The model under review builds one solid part; all positions refer to its coordinate system, in mm. Face numbers are marked on the shaded views. A direction names the side the tool comes from. Give positions to 0.01 mm unless a question says otherwise; leave off trailing zeros. Loops run counter-clockwise (first coordinate to the right, second up) from the corner with the lowest first, then second, coordinate; pieces in that order, holes last. Notation, with made-up numbers: M 76,-31 L 133,-31 A14 cw 133,-23 Z; hole C -5.75,68 d9. An arc over 180 degrees is marked long. Return JSON: item names as keys, results as strings.
Autodesk Inventor part; units mm, degrees
ref_plane "YZ Plane" through (0, 0, 0) normal (1, 0, 0) x (0, 1, 0)
ref_plane "XZ Plane" through (0, 0, 0) normal (0, 1, 0) x (-1, 0, 0)
ref_plane "XY Plane" through (0, 0, 0) normal (0, 0, 1) x (1, 0, 0)
sketch "Sketch1" plane through (0, 0, 0) normal (0, 0, 1) x (1, 0, 0)
  line L0 (0, 0) -> (47, 0)
  line L1 (51, 4) -> (51, 33)
  line L2 (47, 37) -> (0, 37)
  line L3 (0, 37) -> (0, 0)
  circle A0 centre (42, 18.5) radius 4.25
  line L4 (47, 37) -> (51, 33)
  line L5 (47, 0) -> (51, 4)
  line L6 (10, 34) -> (16, 34)
  line L7 (16, 34) -> (16, 26)
  line L8 (16, 26) -> (10, 26)
  line L9 (10, 26) -> (10, 34)
  line L10 (10, 11) -> (16, 11)
  line L11 (16, 11) -> (16, 3)
  line L12 (16, 3) -> (10, 3)
  line L13 (10, 3) -> (10, 11)
  line L14 (10, 26) -> (16, 11) construction
  line L15 (10, 11) -> (16, 26) construction
  circle A1 centre (42, 18.5) radius 16 construction
  line L16 (24, 37) -> (24, 0) construction
  point P0 (51, 37)
  point P1 (51, 0)
  point P2 (0, 18.5)
  point P3 (13, 18.5)
  dimension "d0" = 4
  dimension "d1" = 4
  dimension "d2" = 4
  dimension "d3" = 4
  dimension "d4" = 8.5
  dimension "d5" = 37
  dimension "d6" = 6
  dimension "d7" = 8
  dimension "d8" = 8
  dimension "d9" = 15
  dimension "d10" = 10
  dimension "d11" = 32
  dimension "d12" = 9
  dimension "d13" = 26
  dimension "d14" = 24
extrude "Extrusion1" add sketch "Sketch1" along normal blind 6
sketch "Sketch2" plane through (0, 0, 6) normal (0, 0, 1) x (1, 0, 0)
  line L0 (16, 26) -> (10, 26)
  line L1 (0, 37) -> (0, 0)
  line L2 (0, 34) -> (-4, 34)
  line L3 (-6, 32) -> (-6, 28)
  line L4 (-4, 26) -> (0, 26)
  line L5 (0, 26) -> (0, 34)
  line L6 (0, 11) -> (-4, 11)
  line L7 (-6, 9) -> (-6, 5)
  line L8 (-4, 3) -> (0, 3)
  line L9 (0, 3) -> (0, 11)
  arc A0 (-4, 34) -> (-6, 32) centre (-4, 32) ccw
  arc A1 (-6, 28) -> (-4, 26) centre (-4, 28) ccw
  arc A2 (-4, 11) -> (-6, 9) centre (-4, 9) ccw
  arc A3 (-6, 5) -> (-4, 3) centre (-4, 5) ccw
  dimension "d17" = 2
  dimension "d18" = 6
  dimension "d19" = 8
  dimension "d20" = 8
  dimension "d21" = 15
extrude "Extrusion2" add sketch "Sketch2" against normal blind 6
properties part number "y_carriage_belt_iddler"
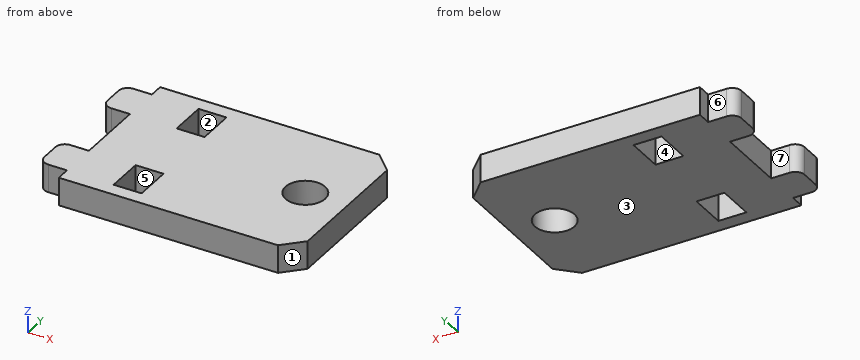
1) Tool access review of the marked faces 5, 6 and 7: name each direction out of +Z, -Z, +X, -X, +Y, -Y from which nothing blocks a thin tool from reaching the whole face with its end or side.
From the geometry:
{"face 5": "+Z, -Z", "face 6": "+Z, -Z, -X, +Y", "face 7": "+Z, -Z, -X"}
2) Consider section D-D on y = 13.5. Write out the cut boundary in (x, z).
From the geometry:
{"outline": "M 0,0 L 51,0 L 51,6 L 0,6 Z"}
3) Insertion check: pin 1 (0.9 mm diameter, centred on y = 1, z = 4, fed in from -X); pin 2 (2.5 mm diameter, centred on y = 35, z = 3.5, fed in from -X); pin 3 (1.2 mm diameter, centred on x = -1.5, z = 3.5, fed in from +Y). Each pin has a flat end and moves straight along its axis. Give the tip position at first contact, or say it passes through.
From the geometry:
{"pin 1": "x = 0", "pin 2": "x = -4.97", "pin 3": "y = 34"}
4) Consider section B-B on z = 5.25. Write out the cut boundary in (x, y).
From the geometry:
{"outline": "M -6,5 A2 ccw -4,3 L 0,3 L 0,0 L 47,0 L 51,4 L 51,33 L 47,37 L 0,37 L 0,34 L -4,34 A2 ccw -6,32 L -6,28 A2 ccw -4,26 L 0,26 L 0,11 L -4,11 A2 ccw -6,9 Z; hole M 10,3 L 16,3 L 16,11 L 10,11 Z; hole M 10,26 L 16,26 L 16,34 L 10,34 Z; hole C 42,18.5 d8.5"}
5) Wall thickness on L1, parallel to Y at x = 42, z = 3.3; L2, parallel to X at y = 14, z = 1.65; L3, parallel to X at y = 19, z = 4: over which ranges is each line inside the solid? List them lowest first. Write a range as from..to.
From the geometry:
{"L1": "0..14.25, 22.75..37", "L2": "0..51", "L3": "0..37.78, 46.22..51"}
6) The part is to be moulded in two halves that separate along X. For the marked faces 1, 2, 3 and 4, say which applies: released by +X, released by -X, zero draft, split by the parting line, or undercut.
From the geometry:
{"face 1": "released by +X", "face 2": "undercut", "face 3": "zero draft", "face 4": "undercut"}
7) Consider section C-C on y = 18.5. Write out the cut boundary in (x, z), then the cut area to 3 significant figures.
From the geometry:
{"outline": "M 0,0 L 37.75,0 L 37.75,6 L 0,6 Z; M 46.25,0 L 51,0 L 51,6 L 46.25,6 Z", "area": "255 mm²"}
8) Consider section A-A on x = 42. Write out the cut boundary in (y, z), then the cut area to 3 significant figures.
From the geometry:
{"outline": "M 0,0 L 14.25,0 L 14.25,6 L 0,6 Z; M 22.75,0 L 37,0 L 37,6 L 22.75,6 Z", "area": "171 mm²"}
